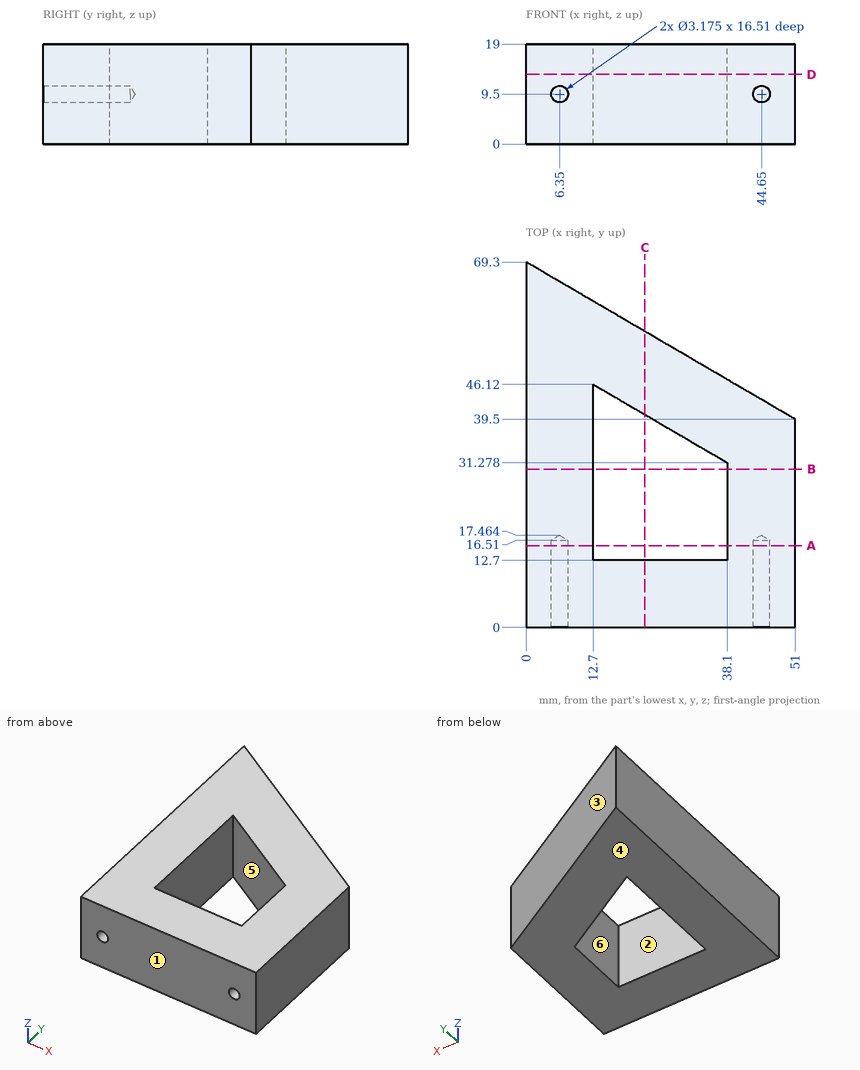
Geometry: see drawing. Coordinates: mm, zero at the bounding-box minimum. A direction names the side the tool comes from. Coordinates: 2 decimals unless noted, no trailing zeros. Order: outer loops, then holes, each group sorted by start corner. A loop starts at its lowest first (then second) coordinate and runs counter-clockwise, first axis right, second up. Notation, with made-up numbers: (18.25, 5.25) - (49.25, 5.25) arc R27 cw to (49.25, 26.25) - close; hole circle Ø7 at (41.5, 67). An arc over 180 degrees is marked (long way). Use one line per item in the form item = value.
1) Set-up query: the marked faces 1 and 2. Return all of +Z, -Z, +X, -X, +Y, -Y with unobstructed straight access to the full face (end or side cutting, diameter ignored); none if empty.
Solutions:
face_1 = +Z, -Z, +X, -X, -Y
face_2 = +Z, -Z
2) Pin query (flat end, axial travel): pin 1 (5 mm diameter, centred on x = 9, z = 13, fed in from +Y); pin 2 (5 mm diameter, centred on x = 44.65, z = 9.5, fed in from +Y); pin 3 (4 mm diameter, centred on y = 45, z = 15.5, fed in from +X). Return the tip coordinate at first contact, or that it passes through.
Solutions:
pin_1 = 65.5
pin_2 = 44.67
pin_3 = 45.01
3) Section D-D (z = 13.25). Return loops of the section in (x, y).
Solutions:
outline = (0, 0) - (51, 0) - (51, 39.5) - (0, 69.3) - close; hole (12.7, 12.7) - (38.1, 12.7) - (38.1, 31.28) - (12.7, 46.12) - close
4) Section B-B (y = 30). Return loops of the section in (x, z).
Solutions:
outline = (0, 0) - (12.7, 0) - (12.7, 19) - (0, 19) - close; (38.1, 0) - (51, 0) - (51, 19) - (38.1, 19) - close
5) Mould query, pull axis Y, two halves, no side actions, for the marked faces 3, 4, 5 and 6. Classes: +Y half, -Y half, draft (parallel to the pull), parting line (faces both ways), or undercut.
Solutions:
face_3 = +Y half
face_4 = draft
face_5 = undercut
face_6 = undercut
6) Ray query, L1, parallel to X at y = 4.25, z = 9.5; L2, parallel to Z at x = 6.35, y = 6.75; L3, parallel to X at y = 18.5, z = 11.75. Return the intervals inside material, ascending.
Solutions:
L1 = 0 to 4.76, 7.94 to 43.06, 46.24 to 51
L2 = 0 to 7.91, 11.09 to 19
L3 = 0 to 12.7, 38.1 to 51
7) Section A-A (y = 15.5). State how many separate pieces and enclosed holes the cut face has.
Solutions:
separate_pieces = 2
enclosed_holes = 2
8) Section C-C (x = 22.5). Return loops of the section in (y, z), then the cut area to 3 significant figures.
Solutions:
outline = (0, 0) - (12.7, 0) - (12.7, 19) - (0, 19) - close; (40.39, 0) - (56.15, 0) - (56.15, 19) - (40.39, 19) - close
area = 541 mm^2
